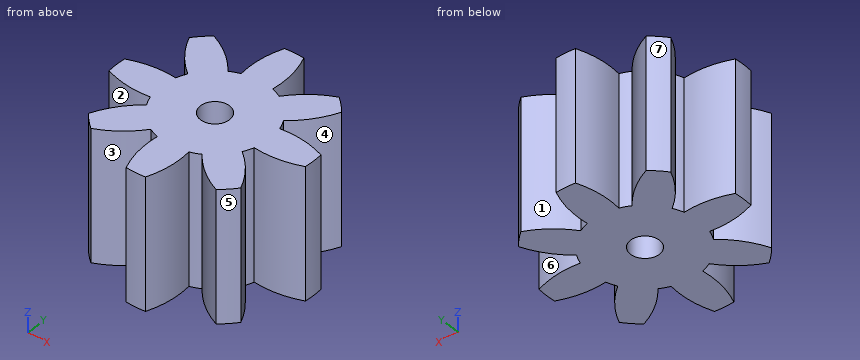
Autodesk Inventor part; units mm, degrees
ref_plane "Work Plane2" through (0, 0, 5) normal (0, 0, 1) x (1, 0, 0)
ref_plane "Work Plane8" through (0, 0, 0) normal (0.9238795, 0.3826834, 0) x (0, 0, 1)
ref_plane "Work Plane9" through (0, 0, 0) normal (1, 0, 0) x (0, 1, 0)
sketch "Sketch1" plane through (0, 0, 0) normal (0, 0, 1) x (1, 0, 0)
  circle A0 centre (0, 0) radius 7.5
  dimension "d0" = 15
extrude "Extrusion1" add sketch "Sketch1" along normal blind 10
ref_plane "Work Plane2" through (0, 0, 5) normal (0, 0, 1) x (1, 0, 0)
sketch "Sketch2" plane through (0, 0, 0) normal (0, 0, -1) x (-1, 0, 0)
  circle A0 centre (0, 0) radius 7.5
  circle A1 centre (0, 0) radius 6
  dimension "d3" = 12
surface extrude "Pitch Diameter" sketch "Sketch2" against normal through all shown no curves A1
ref_plane "Work Plane8" through (0, 0, 0) normal (0.9238795, 0.3826834, 0) x (0, 0, 1)
ref_plane "Work Plane9" through (0, 0, 0) normal (1, 0, 0) x (0, 1, 0)
spur gear teeth "Spur Gear" teeth 8 pitch diameter 12 tip diameter 15 root diameter 8.25 face width 10 start plane through (0, 0, 0) normal (0, 0, -1) x (-1, 0, 0)
sketch "Sketch3" plane through (0, 0, 10) normal (0, 0, 1) x (1, 0, 0)
  arc A0 (-4.7579, 5.7976) -> (-5.7976, 4.7579) centre (0, 0) ccw
  circle A1 centre (0, 0) radius 1.1
  dimension "d49" = 2.2
extrude "Extrusion2" cut sketch "Sketch3" against normal blind 10
equation "\"d0\" = da_da"
equation "\"d1\" = da_b"
equation "\"d3\" = da_dw"
equation "\"d16\" = da_aw"
equation "\"d43\" = da_aw"
equation "\"d46\" = da_aw"
properties part number "Spur Gear1" material "Steel, Alloy"
Input: part model. Units: mm. Frame: model coordinates. Face numbers are marked on the shaded views. A direction names the side the tool comes from. Give positions to 0.01 mm unless a question says otherwise; leave off trailing zeros. Loops run counter-clockwise (first coordinate to the right, second up) from the corner with the lowest first, then second, coordinate; pieces in that order, holes last. Notation, with made-up numbers: (1, 44.25) -> (24, 44.25) arc R21 cw to (24, 76.25) -> close; hole circle Ø11 at (39, 66). An arc over 180 degrees is marked (long way). Answer as a JSON object with one key per item and string values. Group by question number.
Item 1: Line query: probe 1 along Y at (x, z) = (0, 4); probe 2 along X at (y, z) = (4.5, 2.5). Output: solid intervals per line, ascending.
Item 2: Pull-direction query (X, two-part tool) for the marked faces 5, 6 and 7; classes: released by +X, released by -X, zero draft, split by the parting line, or undercut.
Item 3: Cut plane D-D, the plane x = -4.5. Return the cut outline in (y, z), and give its area (3 significant figures).
Item 4: Reachability of the marked faces 1, 2, 3 and 4 from +Z, -Z, +X, -X, +Y, -Y: full face, straight path, thin tool, end or side. Return the list, or none.
Item 5: Pin query (flat end, axial travel): P1, Ø1.5, axis at y = 1, z = 4, coming from the +X side; P2, Ø1, axis at y = 3, z = 8, coming from the -X side; P3, Ø1, axis at y = -2.5, z = 7.5, coming from the +X side. Return the tip coordinate at first contact, or that it passes through.
Item 6: Cut plane A-A, the plane y = 0. Return the cut outline in (x, z), and give its area (3 significant figures).
Checks:
{
 "1": {"probe 1": "y = -7.5 to -1.1, 1.1 to 7.5", "probe 2": "x = -5.68 to -2.74, -1.24 to 1.24, 2.74 to 5.68"},
 "2": {"face 5": "released by +X", "face 6": "undercut", "face 7": "released by -X"},
 "3": {"outline": "(-5.68, 0) -> (-2.74, 0) -> (-2.74, 10) -> (-5.68, 10) -> close; (-1.24, 0) -> (1.24, 0) -> (1.24, 10) -> (-1.24, 10) -> close; (2.74, 0) -> (5.68, 0) -> (5.68, 10) -> (2.74, 10) -> close", "area": "83.8 mm²"},
 "4": {"face 1": "+Z, -Z, +Y", "face 2": "+Z, -Z", "face 3": "+Z, -Z, -Y", "face 4": "+Z, -Z, +X"},
 "5": {"P1": "stops at x = 7.5", "P2": "stops at x = -5.11", "P3": "stops at x = 4.73"},
 "6": {"outline": "(-7.5, 0) -> (-1.1, 0) -> (-1.1, 10) -> (-7.5, 10) -> close; (1.1, 0) -> (7.5, 0) -> (7.5, 10) -> (1.1, 10) -> close", "area": "128 mm²"}
}
